For this review, use the dimensioned drawing (mm, ordinates from the lowest corner) and the shaded views. Round coordinates to 2 decimals unless told otherwise and drop trailing zeros. Loops run counter-clockwise (first coordinate to the right, second up) from the corner with the lowest first, then second, coordinate; pieces in that order, holes last. Notation, with made-up numbers: (64, 63.5) - (116, 63.5) arc R16 cw to (116, 83.5) - close; hole circle Ø3 at (60.5, -6). An arc over 180 degrees is marked (long way). Answer as CSV lines item,"result". Start each with the question number.
(1) Consider section C-C (x = 5). Give the boundary of the cut face in (y, z), and give its area (3 significant figures).
(2) Wall thickness on L1, parallel to Z at x = 2.5, y = 1; L2, parallel to Y at x = 0.75, z = 21; L3, parallel to Y at x = 1, z = 13.5: over which ranges is each line inside the solid? List them lowest first.
(3) Consider section A-A (z = 20.5). Give the boundary of the cut face in (x, y), and give its area (3 significant figures).
(4) For P1, Ø1.5, axis at x = 6.5, z = 23, coming from the +Y side; P2, Ø4, axis at x = 2, y = 3.5, coming from the +Z side; P3, Ø1, axis at y = 5.5, z = 25.5, coming from the -X side; P4, Ø4, axis at x = 3, y = 4.5, coming from the -Z side, all flat-tipped, find the tip position at first contact; note any pin that passes through.
(5) Consider section B-B (z = 3.5). Give the boundary of the cut face in (x, y), and give its area (3 significant figures).
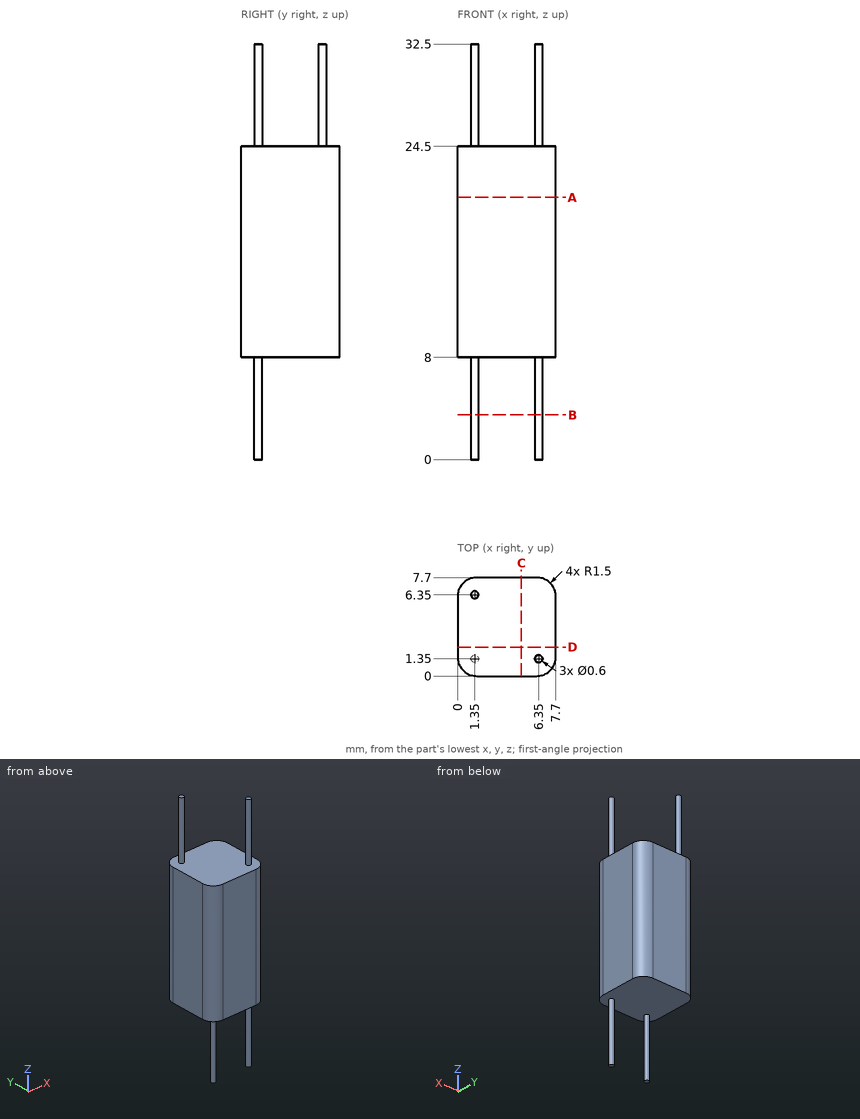
Determined:
1,outline,"(0, 8) - (7.7, 8) - (7.7, 24.5) - (0, 24.5) - close"
1,area,"127 mm^2"
2,L1,"z = 8 to 24.5"
2,L2,"y = 0.2 to 7.5"
2,L3,"y = 0.09 to 7.61"
3,outline,"(0, 1.5) arc R1.5 ccw to (1.5, 0) - (6.2, 0) arc R1.5 ccw to (7.7, 1.5) - (7.7, 6.2) arc R1.5 ccw to (6.2, 7.7) - (1.5, 7.7) arc R1.5 ccw to (0, 6.2) - close"
3,area,"57.4 mm^2"
4,P1,"stops at y = 7.7"
4,P2,"stops at z = 24.5"
4,P3,"passes through"
4,P4,"stops at z = 8"
5,outline,"circle Ø0.6 at (1.35, 1.35); circle Ø0.6 at (6.35, 1.35)"
5,area,"0.565 mm^2"
